Geometry: final body of the model. Coordinates: model frame, mm. A direction names the side the tool comes from. Round coordinates to 2 decimals unless told otherwise and drop trailing zeros. Write each loop counter-clockwise with the first axis right and the second up, starting at its lowest first coordinate (ties: lowest second). Pieces come first, ordered by that corner, then holes. Notation, with made-up numbers: M 7,21 L 20,21 A26 ccw 20,53 Z; hole C 27,-13 d11. An arc over 180 degrees is marked long. Use one line per item in the form item = value. Start each with the question number.
from build123d import *

# Parameters (mm, degrees)
SKETCH1_R           = 10.91
BOSS_EXTRUDE1_DEPTH = 10.91


with BuildPart() as part:
    # Sketch1 → Boss-Extrude1 (new body)
    with BuildSketch(Plane(origin=(0, 0, 0), x_dir=(1, 0, 0), z_dir=(0, 1, 0))):
        with BuildLine():
            Line((0, -5.455), (0, 5.455))
            Line((0, 5.455), (23.281662845, 5.455))
            ThreePointArc((23.281662845, 5.455), (32.73, 10.91), (42.178337155, 5.455))
            Line((42.178337155, 5.455), (65.222277444, 5.455))
            ThreePointArc((65.222277444, 5.455), (64.890066177, 8.542939281), (64.411740124, 11.611642185))
            Line((64.411740124, 11.611642185), (53.873489359, 8.787926403))
            ThreePointArc((53.873489359, 8.787926403), (47.192506085, 12.645193894), (51.049773577, 19.326177168))
            Line((51.049773577, 19.326177168), (61.588024342, 22.14989295))
            ThreePointArc((61.588024342, 22.14989295), (56.681362678, 32.725), (49.976382157, 42.261847174))
            Line((49.976382157, 42.261847174), (42.261847174, 34.547312191))
            ThreePointArc((42.261847174, 34.547312191), (34.547312191, 34.547312191), (34.547312191, 42.261847174))
            Line((34.547312191, 42.261847174), (42.261847174, 49.976382157))
            ThreePointArc((42.261847174, 49.976382157), (32.725, 56.681362678), (22.14989295, 61.588024342))
            Line((22.14989295, 61.588024342), (19.326177168, 51.049773577))
            ThreePointArc((19.326177168, 51.049773577), (12.645193894, 47.192506085), (8.787926403, 53.873489359))
            Line((8.787926403, 53.873489359), (11.611642185, 64.411740124))
            ThreePointArc((11.611642185, 64.411740124), (0, 65.45), (-11.611642185, 64.411740124))
            Line((-11.611642185, 64.411740124), (-8.787926403, 53.873489359))
            ThreePointArc((-8.787926403, 53.873489359), (-12.645193894, 47.192506085), (-19.326177168, 51.049773577))
            Line((-19.326177168, 51.049773577), (-22.14989295, 61.588024342))
            ThreePointArc((-22.14989295, 61.588024342), (-32.725, 56.681362678), (-42.261847174, 49.976382157))
            Line((-42.261847174, 49.976382157), (-34.547312191, 42.261847174))
            ThreePointArc((-34.547312191, 42.261847174), (-34.547312191, 34.547312191), (-42.261847174, 34.547312191))
            Line((-42.261847174, 34.547312191), (-49.976382157, 42.261847174))
            ThreePointArc((-49.976382157, 42.261847174), (-56.681362678, 32.725), (-61.588024342, 22.14989295))
            Line((-61.588024342, 22.14989295), (-51.049773577, 19.326177168))
            ThreePointArc((-51.049773577, 19.326177168), (-47.192506085, 12.645193894), (-53.873489359, 8.787926403))
            Line((-53.873489359, 8.787926403), (-64.411740124, 11.611642185))
            ThreePointArc((-64.411740124, 11.611642185), (-65.45, 0), (-64.411740124, -11.611642185))
            Line((-64.411740124, -11.611642185), (-53.873489359, -8.787926403))
            ThreePointArc((-53.873489359, -8.787926403), (-47.192506085, -12.645193894), (-51.049773577, -19.326177168))
            Line((-51.049773577, -19.326177168), (-61.588024342, -22.14989295))
            ThreePointArc((-61.588024342, -22.14989295), (-56.681362678, -32.725), (-49.976382157, -42.261847174))
            Line((-49.976382157, -42.261847174), (-42.261847174, -34.547312191))
            ThreePointArc((-42.261847174, -34.547312191), (-34.547312191, -34.547312191), (-34.547312191, -42.261847174))
            Line((-34.547312191, -42.261847174), (-42.261847174, -49.976382157))
            ThreePointArc((-42.261847174, -49.976382157), (-32.725, -56.681362678), (-22.14989295, -61.588024342))
            Line((-22.14989295, -61.588024342), (-19.326177168, -51.049773577))
            ThreePointArc((-19.326177168, -51.049773577), (-12.645193894, -47.192506085), (-8.787926403, -53.873489359))
            Line((-8.787926403, -53.873489359), (-11.611642185, -64.411740124))
            ThreePointArc((-11.611642185, -64.411740124), (0, -65.45), (11.611642185, -64.411740124))
            Line((11.611642185, -64.411740124), (8.787926403, -53.873489359))
            ThreePointArc((8.787926403, -53.873489359), (12.645193894, -47.192506085), (19.326177168, -51.049773577))
            Line((19.326177168, -51.049773577), (22.14989295, -61.588024342))
            ThreePointArc((22.14989295, -61.588024342), (32.725, -56.681362678), (42.261847174, -49.976382157))
            Line((42.261847174, -49.976382157), (34.547312191, -42.261847174))
            ThreePointArc((34.547312191, -42.261847174), (34.547312191, -34.547312191), (42.261847174, -34.547312191))
            Line((42.261847174, -34.547312191), (49.976382157, -42.261847174))
            ThreePointArc((49.976382157, -42.261847174), (56.681362678, -32.725), (61.588024342, -22.14989295))
            Line((61.588024342, -22.14989295), (51.049773577, -19.326177168))
            ThreePointArc((51.049773577, -19.326177168), (47.192506085, -12.645193894), (53.873489359, -8.787926403))
            Line((53.873489359, -8.787926403), (64.411740124, -11.611642185))
            ThreePointArc((64.411740124, -11.611642185), (64.890066177, -8.542939281), (65.222277444, -5.455))
            Line((65.222277444, -5.455), (42.178337155, -5.455))
            ThreePointArc((42.178337155, -5.455), (33.295026603, -10.895358871), (23.896615512, -6.403078828))
            Line((23.896615512, -6.403078828), (20.358337155, -5.455))
            Line((20.358337155, -5.455), (0, -5.455))
        make_face()
        with Locations(Location((-16.365, -28.345011466, 0), (0, 0, 270))):
            Circle(SKETCH1_R, mode=Mode.SUBTRACT)
        with Locations(Location((16.365, -28.345011466, 0), (0, 0, 270))):
            Circle(SKETCH1_R, mode=Mode.SUBTRACT)
        with Locations(Location((-32.73, 0, 0), (0, 0, 270))):
            Circle(SKETCH1_R, mode=Mode.SUBTRACT)
        with Locations(Location((-16.365, 28.345011466, 0), (0, 0, 270))):
            Circle(SKETCH1_R, mode=Mode.SUBTRACT)
        with Locations(Location((16.365, 28.345011466, 0), (0, 0, 270))):
            Circle(SKETCH1_R, mode=Mode.SUBTRACT)
    extrude(amount=BOSS_EXTRUDE1_DEPTH)


solid = part.part
1. Set-up query: faces 1 (the face through (-59.07, 5.38, -10.18)), 2 (the face through (64.896, 5.379, -8.5)), 3 (the face through (56.393, 5.379, 20.758)), 4 (the face through (-56.25, 5.38, 20.72)), 5 (the face through (-20.72, 5.38, -56.25)). Return all of +Z, -Z, +X, -X, +Y, -Y with unobstructed straight access to the full face (end or side cutting, diameter ignored); none if empty.
2. Contact query for flat-ended pins moving along their axis: pin 1 (2 mm diameter, centred on x = -16.5, y = 1.5, fed in from -Z); pin 2 (1 mm diameter, centred on y = 7.5, z = 46.5, fed in from +X); pin 3 (6 mm diameter, centred on y = 8, z = 26, fed in from -X); pin 4 (17.5 mm diameter, centred on x = 16.36, z = -28.35, fed in from -Y). Output: stop coordinate, or through.
3. Section query C-C (y = 1.75). Give the number of separate pieces and of enclosed holes in the cut face, then the cut area to 3 significant figures.
4. Section query A-A (z = 0). Return loops of the section in (x, y), then the cut area to 3 significant figures.
5. Ray query, probe 1 along X at (y, z) = (2, 29.5); probe 2 along Z at (x, y) = (-36, 6.75); probe 3 along Z at (x, y) = (8.5, 6.5) (3 decimals). Return the intervals inside material, ascending.
6. Section query B-B (x = -38). Return loops of the section in (y, z), then the cut area to 3 significant figures.
Checks:
q1.face_1 = +Y, -Y
q1.face_2 = -Z, +X, +Y, -Y
q1.face_3 = +X, +Y, -Y
q1.face_4 = -X, +Y, -Y
q1.face_5 = -Z, +Y, -Y
q2.pin_1 = -48.23
q2.pin_2 = 39.29
q2.pin_3 = -61.28
q2.pin_4 = through
q3.separate_pieces = 1
q3.enclosed_holes = 5
q3.area = 8,720 mm^2
q4.outline = M -65.45,0 L -43.64,0 L -43.64,10.91 L -65.45,10.91 Z; M -21.82,0 L 0,0 L 0,10.91 L -21.82,10.91 Z
q4.area = 476 mm^2
q5.probe_1 = -58.42 to -27.21, -5.52 to 5.52, 27.21 to 58.42
q5.probe_2 = -54.66 to -43.71, -33.51 to -10.41, 10.41 to 33.51, 43.71 to 54.66
q5.probe_3 = -64.896 to -35.906, -20.784 to -5.455, 5.455 to 20.784, 35.906 to 64.896
q6.outline = M 0,-53.29 L 10.91,-53.29 L 10.91,-45.71 L 0,-45.71 Z; M 0,-32.96 L 10.91,-32.96 L 10.91,-9.55 L 0,-9.55 Z; M 0,9.55 L 10.91,9.55 L 10.91,32.96 L 0,32.96 Z; M 0,45.71 L 10.91,45.71 L 10.91,53.29 L 0,53.29 Z
q6.area = 676 mm^2
